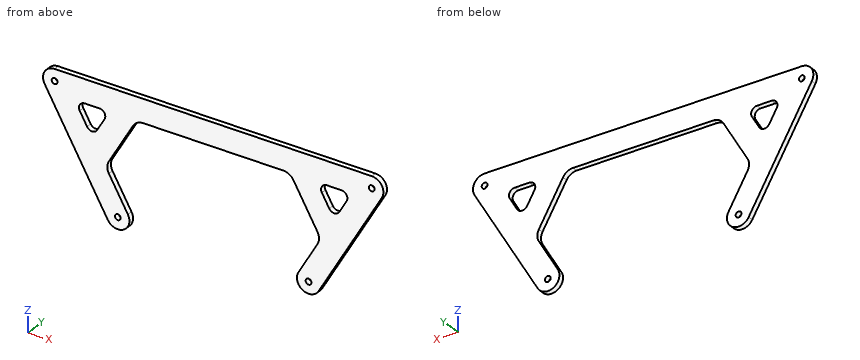
```python
from build123d import *

# Parameters (mm, degrees)
SKETCH1_R           = 3.175
BOSS_EXTRUDE1_DEPTH = 5.842
FILLET1_R           = 6.35
FILLET2_R           = 12.7


with BuildPart() as part:
    # Sketch1 → Boss-Extrude1 (new body)
    with BuildSketch(Plane(origin=(0, 0, 0), x_dir=(1, 0, 0), z_dir=(0, 1, 0))):
        with BuildLine():
            Line((-115.350561828, 126.131830356), (-184.506633828, 6.35))
            ThreePointArc((-184.506633828, 6.35), (-184.506633828, -6.35), (-173.5081112, -12.7))
            Line((-173.5081112, -12.7), (173.5081112, -12.7))
            ThreePointArc((173.5081112, -12.7), (184.506633828, -6.35), (184.506633828, 6.35))
            Line((184.506633828, 6.35), (115.350561828, 126.131830356))
            ThreePointArc((115.350561828, 126.131830356), (98.0020392, 130.780352984), (93.353516572, 113.431830356))
            Line((93.353516572, 113.431830356), (117.796369106, 71.095567884))
            Line((117.796369106, 71.095567884), (84.081672269, 12.7))
            Line((84.081672269, 12.7), (-84.081672269, 12.7))
            Line((-84.081672269, 12.7), (-117.796369106, 71.095567884))
            Line((-117.796369106, 71.095567884), (-93.353516572, 113.431830356))
            ThreePointArc((-93.353516572, 113.431830356), (-98.0020392, 130.780352984), (-115.350561828, 126.131830356))
        make_face()
        with Locations(Location((-173.5081112, 0, 0), (0, 0, 270))):
            Circle(SKETCH1_R, mode=Mode.SUBTRACT)
        with Locations(Location((-104.3520392, 119.781830356, 0), (0, 0, 270))):
            Circle(SKETCH1_R, mode=Mode.SUBTRACT)
        with Locations(Location((104.3520392, 119.781830356, 0), (0, 0, 90))):
            Circle(SKETCH1_R, mode=Mode.SUBTRACT)
        with Locations(Location((173.5081112, 0, 0), (0, 0, 90))):
            Circle(SKETCH1_R, mode=Mode.SUBTRACT)
        Polygon((151.511065944, 12.7), (113.411065944, 12.7), (132.461065944, 45.695567884), align=None, mode=Mode.SUBTRACT)
        Polygon((-132.461065944, 45.695567884), (-113.411065944, 12.7), (-151.511065944, 12.7), align=None, mode=Mode.SUBTRACT)
    extrude(amount=BOSS_EXTRUDE1_DEPTH)

    # Fillet1
    fillet1_edges = [part.edges().sort_by_distance(p)[0] for p in [
        (151.511065944, 2.921, -12.7),
        (132.461065944, 2.921, -45.695567884),
        (113.411065944, 2.921, -12.7),
        (-132.461065944, 2.921, -45.695567884),
        (-151.511065944, 2.921, -12.7),
        (-113.411065944, 2.921, -12.7),
    ]]
    fillet(fillet1_edges, radius=FILLET1_R)

    # Fillet2
    fillet2_edges = [part.edges().sort_by_distance(p)[0] for p in [
        (-117.796369106, 2.921, -71.095567884),
        (-84.081672269, 2.921, -12.7),
        (84.081672269, 2.921, -12.7),
        (117.796369106, 2.921, -71.095567884),
    ]]
    fillet(fillet2_edges, radius=FILLET2_R)


solid = part.part
```
Source: CAD feature listing. Evaluate the final solid. Frame: model axes, mm. Give positions to 0.01 mm unless a question says otherwise; leave off trailing zeros. Loops run counter-clockwise (first coordinate to the right, second up) from the corner with the lowest first, then second, coordinate; pieces in that order, holes last. Notation, with made-up numbers: M 8.5,83 L 58.5,83 A30 ccw 58.5,119 Z; hole C 76,71.5 d7. An arc over 180 degrees is marked long. Put each result on its own line as item: value.
Q1. Line query: probe 1 along X at (y, z) = (3.15, 0); probe 2 along Z at (x, y) = (77.5, 1.45); probe 3 along Z at (x, y) = (104.5, 2.8). Output: solid intervals per line, ascending. Write a range as [from, to].
Response values:
probe 1: x = [-186.21, -176.68], [-170.33, 170.33], [176.68, 186.21]
probe 2: z = [-12.72, 12.7]
probe 3: z = [-132.48, -122.95], [-116.61, -94.13], [-48.07, 12.7]
Q2. Section A-A (z = -105.5). Return the cut outline in (x, y).
Response values:
outline: M -127.26,0 L -97.93,0 L -97.93,5.84 L -127.26,5.84 Z; M 97.93,0 L 127.26,0 L 127.26,5.84 L 97.93,5.84 Z
Q3. Section C-C (x = -43). Return the cut outline in (y, z), and give its area (3 significant figures).
Response values:
outline: M 0,-12.7 L 5.84,-12.7 L 5.84,12.7 L 0,12.7 Z
area: 148 mm²
Q4. Pin query (flat end, axial travel): P1, Ø1, axis at x = -37.5, y = 2, coming from the -Z side; P2, Ø1.5, axis at y = 3.5, z = -93.5, coming from the -X side; P3, Ø1, axis at y = 3, z = -108, coming from the +X side. Return the tip coordinate at first contact, or that it passes through.
Response values:
P1: stops at z = -12.7
P2: stops at x = -134.62
P3: stops at x = 126.11
Q5. Section B-B (y = 3.5). Count the separate pieces of the cut face and the enclosed holes in it, and give its area (3 significant figures).
Response values:
separate pieces: 1
enclosed holes: 6
area: 18,900 mm²
